```python
from build123d import *

# Parameters (mm, degrees)
SKETCH1_R           = 1.525
BOSS_EXTRUDE1_DEPTH = 3
SKETCH2_W           = 80
SKETCH2_H           = 35
CUT_EXTRUDE1_DEPTH  = 5
SKETCH4_R           = 1.55
CUT_EXTRUDE2_DEPTH  = 277.097497981


with BuildPart() as part:
    # Sketch1 → Boss-Extrude1 (new body)
    with BuildSketch(Plane(origin=(0, 3, 0), x_dir=(1, 0, 0), z_dir=(0, 1, 0))):
        with BuildLine():
            Line((200.301843205, 35), (200.301843205, 155))
            ThreePointArc((200.301843205, 155), (197.372911017, 162.071067812), (190.301843205, 165))
            Line((190.301843205, 165), (40.301843205, 165))
            Line((40.301843205, 165), (40.301843205, 190))
            ThreePointArc((40.301843205, 190), (0.301843205, 95), (40.301843205, 0))
            Line((40.301843205, 0), (40.301843205, 25))
            Line((40.301843205, 25), (190.301843205, 25))
            ThreePointArc((190.301843205, 25), (197.372911017, 27.928932188), (200.301843205, 35))
        make_face()
        with Locations(Location((80.301843205, 33.16, 0), (0, 0, 90))):
            Circle(SKETCH1_R, mode=Mode.SUBTRACT)
        with Locations(Location((80.301843205, 125.09, 0), (0, 0, 90))):
            Circle(SKETCH1_R, mode=Mode.SUBTRACT)
        with Locations(Location((80.301843205, 131.44, 0), (0, 0, 90))):
            Circle(SKETCH1_R, mode=Mode.SUBTRACT)
        with Locations(Location((80.301843205, 137.79, 0), (0, 0, 90))):
            Circle(SKETCH1_R, mode=Mode.SUBTRACT)
        with Locations(Location((80.301843205, 64.91, 0), (0, 0, 90))):
            Circle(SKETCH1_R, mode=Mode.SUBTRACT)
        with Locations(Location((80.301843205, 156.84, 0), (0, 0, 90))):
            Circle(SKETCH1_R, mode=Mode.SUBTRACT)
        with Locations(Location((80.301843205, 150.49, 0), (0, 0, 90))):
            Circle(SKETCH1_R, mode=Mode.SUBTRACT)
        with Locations(Location((80.301843205, 144.14, 0), (0, 0, 90))):
            Circle(SKETCH1_R, mode=Mode.SUBTRACT)
        with Locations(Location((80.301843205, 58.56, 0), (0, 0, 90))):
            Circle(SKETCH1_R, mode=Mode.SUBTRACT)
        with Locations(Location((80.301843205, 52.21, 0), (0, 0, 90))):
            Circle(SKETCH1_R, mode=Mode.SUBTRACT)
        with Locations(Location((80.301843205, 45.86, 0), (0, 0, 90))):
            Circle(SKETCH1_R, mode=Mode.SUBTRACT)
        with Locations(Location((80.301843205, 39.51, 0), (0, 0, 90))):
            Circle(SKETCH1_R, mode=Mode.SUBTRACT)
    extrude(amount=-BOSS_EXTRUDE1_DEPTH)

    # Sketch2 → Cut-Extrude1 (cut)
    with BuildSketch(Plane(origin=(0, 3, 0), x_dir=(1, 0, 0), z_dir=(0, 1, 0))):
        with Locations((160.301843205, 95)):
            Rectangle(SKETCH2_W, SKETCH2_H)
    extrude(amount=-CUT_EXTRUDE1_DEPTH, mode=Mode.SUBTRACT)

    # Sketch4 → Cut-Extrude2 (cut, through all)
    with BuildSketch(Plane(origin=(0, 3, 0), x_dir=(1, 0, 0), z_dir=(0, 1, 0))):
        with Locations(Location((34.819271837, 155.2, 0), (0, 0, 270))):
            Circle(SKETCH4_R)
        with Locations(Location((33.619271837, 106.15, 0), (0, 0, 270))):
            Circle(SKETCH4_R)
        with Locations(Location((110.019271837, 155.2, 0), (0, 0, 270))):
            Circle(SKETCH4_R)
        with Locations(Location((116.269271837, 106.15, 0), (0, 0, 270))):
            Circle(SKETCH4_R)
    extrude(amount=-CUT_EXTRUDE2_DEPTH, mode=Mode.SUBTRACT)


solid = part.part
```
The model under review builds one solid part; all positions refer to its coordinate system, in mm. Round coordinates to 2 decimals unless told otherwise and drop trailing zeros. Write each loop counter-clockwise with the first axis right and the second up, starting at its lowest first coordinate (ties: lowest second). Pieces come first, ordered by that corner, then holes. Notation, with made-up numbers: (79, 85) -> (97, 85) arc R11 ccw to (97, 103) -> close; hole circle Ø4 at (27, 55.25). An arc over 180 degrees is marked (long way). Use CSV: the item, a comma, the result in double quotes.
Q1. Consider section C-C (z = -90.5). Give the boundary of the cut face in (x, y).
Checks:
outline,"(0.38, 0) -> (120.3, 0) -> (120.3, 3) -> (0.38, 3) -> close"
Q2. To check wall thickness, follow probe 1 along Z at (x, y) = (180.5, 0.55); probe 2 along X at (y, z) = (2.3, -106.15); probe 3 along X at (y, z) = (0.95, -155.2). State the ranges of each line that lie inside material, in increasing order. Write a range as [from, to].
Checks:
probe 1,"[-165, -112.5], [-77.5, -25]"
probe 2,"[0.77, 32.07], [35.17, 114.72], [117.82, 120.3]"
probe 3,"[14.73, 33.27], [36.37, 108.47], [111.57, 200.3]"
Q3. For pin 1 Ø4 at (x, z) = (80.3, -45.86) entering from +Y; pin 2 Ø1.5 at (y, z) = (1, -100.5) entering from +X; pin 3 Ø1.5 at (x, y) = (32, 2) entering from -Z; pin 4 Ø0.9 at (x, y) = (147, 2) entering from +Z, all flat-tipped, find the tip position at first contact; note any pin that passes through.
Checks:
pin 1,"y = 3"
pin 2,"x = 120.3"
pin 3,"z = -181.98"
pin 4,"z = -25"
Q4. Consider section B-B (x = 70). Give the boundary of the cut face in (y, z).
Checks:
outline,"(0, -165) -> (3, -165) -> (3, -25) -> (0, -25) -> close"
Q5. Consider section A-A (y = 0.65). State how many separate pieces and enclosed holes the cut face has, then the cut area to 3 significant figures.
Checks:
separate pieces,"1"
enclosed holes,"16"
area,"24,700 mm²"
